```python
from build123d import *

# Parameters (mm, degrees)
F0_W      = 92
F0_H      = 92
F0_W_2    = 88
F0_H_2    = 88
F1_DEPTH  = 92
F2_W      = 6
F2_H      = 1.459
F2_H_2    = 0.7295
F7_DEPTH  = 5
F8_W      = 10
F8_H      = 7.6772981499
F9_DEPTH  = 3
F10_SIZE  = 0.75
F12_COUNT = 4


with BuildPart() as f1:
    # F0 (on Front) → F1 (new body)
    with BuildSketch(Plane.XZ):
        Rectangle(F0_W, F0_H)
        Rectangle(F0_W_2, F0_H_2, mode=Mode.SUBTRACT)
    extrude(amount=F1_DEPTH)

    # F6: sweep along a path in F5
    with BuildLine(Plane(origin=(-33.1, 0, 0), x_dir=(0, -1, 0), z_dir=(-1, 0, 0))) as f6_path:
        Line((84.0388506204, 44), (75.6127773806, 38.1))
    # F2 (on face) → F6 (sweep)
    with BuildSketch(Plane(origin=(0, 0, 44), x_dir=(1, 0, 0), z_dir=(0, 0, -1))):
        with Locations((-33.1, 83.3093506204)):
            Rectangle(F2_W, F2_H)
        with Locations((-33.1, 48.63525)):
            Rectangle(F2_W, F2_H_2)
        with Locations((-33.1, 49.36475)):
            Rectangle(F2_W, F2_H_2)
        with Locations((-33.1, 14.6906493796)):
            Rectangle(F2_W, F2_H)
    sweep(path=f6_path.line)

    # F5 (on line) → F7 (join, symmetric)
    with BuildSketch(Plane(origin=(-33.1, 0, 0), x_dir=(0, -1, 0), z_dir=(-1, 0, 0))):
        Polygon((75.6127773806, 38.1), (77.7549993907, 39.6), (0, 39.6), (0, 38.1), align=None)
    extrude(amount=F7_DEPTH, both=True)

    # F8 (on face) → F9 (cut)
    with BuildSketch(Plane(origin=(0, 0, 38.1), x_dir=(1, 0, 0), z_dir=(0, 0, -1))):
        Polygon((-38.1, 74.8987033772), (-36.1, 77.7549993907), (-38.1, 77.7549993907), align=None)
        Polygon((-30.1, 77.7549993907), (-28.1, 74.8987033772), (-28.1, 77.7549993907), align=None)
        with Locations((-33.1, 3.838649075)):
            Rectangle(F8_W, F8_H)
    extrude(amount=-F9_DEPTH, mode=Mode.SUBTRACT)

    # F10
    f10_edges = [f1.edges().sort_by_distance(p)[0] for p in [
        (-38.1, -41.288001, 38.1),
        (-28.1, -41.288001, 38.1),
    ]]
    chamfer(f10_edges, length=F10_SIZE)

    # F11: F1 across plane


with BuildPart() as f1_1:
    add(f1.part)
    add(f1.part.mirror(Plane.YZ))

    # F12: F1 ×4 about axis
    f12_axis = Axis((0, -46, 0), (0, -1, 0))


with BuildPart() as f1_2:
    add(f1_1.part)
    for i in range(1, F12_COUNT):
        add(f1_1.part.rotate(f12_axis, i * 360 / F12_COUNT))


solid = f1_2.part
```
Read the model definition and answer for the solid it produces. Units are mm, in the model's axes. A direction names the side the tool comes from. Give positions to 0.01 mm unless a question says otherwise; leave off trailing zeros. Order: outer loops, then holes, each group sorted by start corner. A loop starts at its lowest first (then second) coordinate and runs counter-clockwise, first axis right, second up. Notation, with made-up numbers: (-22.5, -15) -> (34.5, -15) arc R31 ccw to (34.5, 15) -> close; hole circle Ø8 at (26.5, 37). An arc over 180 degrees is marked (long way). Write item = value, one per line.
1. A cutting plane is placed at A-A, the plane z = 31.5. Count the separate pieces of the cut face and the enclosed holes in it, and give its area (3 significant figures).
Numbers:
separate_pieces = 2
enclosed_holes = 4
area = 614 mm²
2. Straight lines are drawn through the part: line 1 along Z through (x, y) = (39, -17); line 2 along Z through (x, y) = (-2, -8.5). For each, find the intervals that lie inside material, in ascending order.
Numbers:
line_1 = -46 to -44, -38.1 to -28.1, 28.1 to 38.1, 44 to 46
line_2 = -46 to -44, 44 to 46
3. For faces 4 (the face through (-1, -45, -46)), 5 (the face through (-41.769, -46.544, 33.058)), 6 (the face through (-30.1, -12, -42)), determine the directions among +Z, -Z, +X, -X, +Y, -Y from which every point of the face is accessible in a straight line to the end or side of a thin tool.
Numbers:
face_4 = -Z, +X, -X, +Y, -Y
face_5 = none
face_6 = +Y, -Y
4. A cutting plane is placed at D-D, the plane y = -5.5. Write down the section's boundary in (x, z).
Numbers:
outline = (-46, -46) -> (46, -46) -> (46, 46) -> (-46, 46) -> close; hole (-44, -44) -> (44, -44) -> (44, 44) -> (-44, 44) -> close
5. A cutting plane is placed at C-C, the plane x = -10. Write down the section's boundary in (y, z).
Numbers:
outline = (-92, -46) -> (0, -46) -> (0, -44) -> (-92, -44) -> close; (-92, 44) -> (0, 44) -> (0, 46) -> (-92, 46) -> close
6. The mould has two halves that part along X. Classify faces 1 (the face through (-45, 0, 0)), 2 (the face through (-33, -41, 38.1)), 3 (the face through (46, -45, -1)): +X half, -X half, draft (parallel to the pull), parting line (faces both ways), or undercut.
Numbers:
face_1 = draft
face_2 = undercut
face_3 = +X half
7. Given pin 1 (1.6 mm diameter, centred on x = 35.5, z = -39, fed in from +Y), flat-ended and moving along its own axis, determine where the tip first touches the part or whether it passes through.
Numbers:
pin_1 = -7.68
